Could you check a few things on this drawing? It's one solid part, dimensions in mm from its lowest x, y, z. Coordinates: 2 decimals unless noted, no trailing zeros. Write each loop counter-clockwise with the first axis right and the second up, starting at its lowest first coordinate (ties: lowest second). Pieces come first, ordered by that corner, then holes.
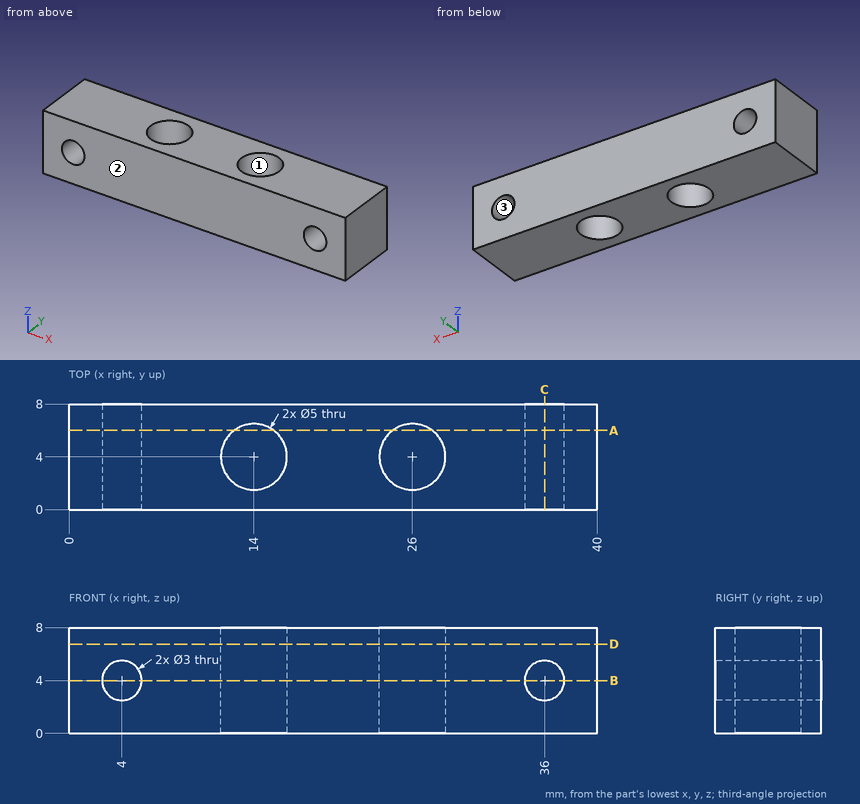
1) We'd pull the mould along Y, two halves only. Please class the marked faces 1, 2 and 3: pulls with the +Y half, pulls with the -Y half, needs draft (parallel to the pull), parting line crosses it, or undercut.
Values follow:
face 1: undercut
face 2: pulls with the -Y half
face 3: needs draft
2) Will this pin go through, and if not, where does the flat tip stop? pin 1 (4 mm diameter, centred on y = 5.5, z = 6, fed in from -X).
Values follow:
pin 1: stops at x = 0
3) Imagine slicing it at A-A on y = 6. Please give me the cut outline in (x, z).
Values follow:
outline: (0, 0) - (12.5, 0) - (12.5, 8) - (0, 8) - close; (15.5, 0) - (24.5, 0) - (24.5, 8) - (15.5, 8) - close; (27.5, 0) - (40, 0) - (40, 8) - (27.5, 8) - close; hole circle Ø3 at (4, 4); hole circle Ø3 at (36, 4)
4) Imagine slicing it at C-C on x = 36. Please give me the cut outline in (y, z), then the cut area to 3 significant figures.
Values follow:
outline: (0, 0) - (8, 0) - (8, 2.5) - (0, 2.5) - close; (0, 5.5) - (8, 5.5) - (8, 8) - (0, 8) - close
area: 40.0 mm2
5) Imagine slicing it at D-D on z = 6.75. Please give me the cut outline in (x, y), then the cut area to 3 significant figures.
Values follow:
outline: (0, 0) - (40, 0) - (40, 8) - (0, 8) - close; hole circle Ø5 at (14, 4); hole circle Ø5 at (26, 4)
area: 281 mm2
6) I need wall thicknesses on probe 1 along Y at (x, z) = (24, 1); probe 2 along Y at (x, z) = (14, 6.75). Which ranges of each line are inside material? Lowest first, please.
Values follow:
probe 1: y = 0 to 2.5, 5.5 to 8
probe 2: y = 0 to 1.5, 6.5 to 8
7) Imagine slicing it at B-B on z = 4. Please give me the cut outline in (x, y).
Values follow:
outline: (0, 0) - (2.5, 0) - (2.5, 8) - (0, 8) - close; (5.5, 0) - (34.5, 0) - (34.5, 8) - (5.5, 8) - close; (37.5, 0) - (40, 0) - (40, 8) - (37.5, 8) - close; hole circle Ø5 at (14, 4); hole circle Ø5 at (26, 4)
